Geometry: final body of the model. Coordinates: model frame, mm. Face numbers are marked on the shaded views. A direction names the side the tool comes from. Coordinates: 2 decimals unless noted, no trailing zeros. Order: outer loops, then holes, each group sorted by start corner. A loop starts at its lowest first (then second) coordinate and runs counter-clockwise, first axis right, second up. Notation, with made-up numbers: (15, 42) - (24, 42) arc R15 cw to (24, 65) - close; hole circle Ø4 at (-2, 85.5). An arc over 180 degrees is marked (long way). Use one line per item in the form item = value. Start each with the question number.
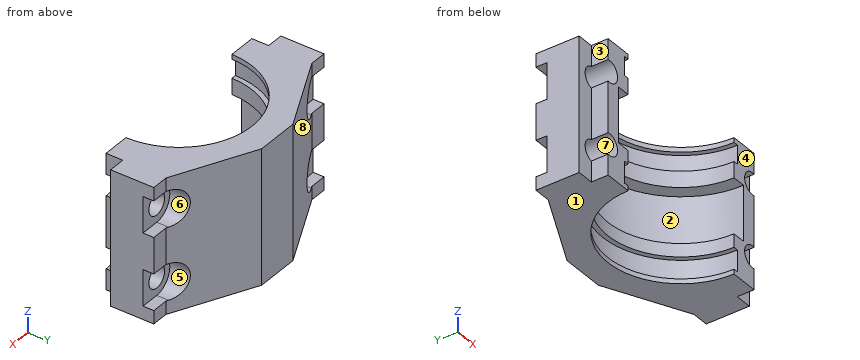
```python
from build123d import *

# Parameters (mm, degrees)
Y_KSEKLIK_EKSTR_ZYON1_DEPTH = 28
KES_EKSTR_ZYON1_DEPTH       = 7.81
KES_EKSTR_ZYON2_DEPTH       = 23
KES_EKSTR_ZYON3_DEPTH       = 9
KES_EKSTR_ZYON4_DEPTH       = 9
KES_EKSTR_ZYON5_DEPTH       = 4.5
IZIM7_R                     = 4.5
KES_EKSTR_ZYON6_DEPTH       = 21.5


with BuildPart() as part:
    # izim1 → Y_kseklik-Ekstr_zyon1 (new body, symmetric)
    with BuildSketch(Plane.XY):
        with BuildLine():
            Line((9, 0), (-9, 0))
            Line((-9, 0), (-42, -16))
            Line((-42, -16), (-49, -16))
            Line((-49, -16), (-49, -34))
            Line((-49, -34), (-42, -34))
            Line((-42, -34), (-42, -41))
            Line((-42, -41), (-30.5, -41))
            ThreePointArc((-30.5, -41), (0, -10.5), (30.5, -41))
            Line((30.5, -41), (42, -41))
            Line((42, -41), (42, -34))
            Line((42, -34), (49, -34))
            Line((49, -34), (49, -16))
            Line((49, -16), (42, -16))
            Line((42, -16), (9, 0))
        make_face()
    extrude(amount=Y_KSEKLIK_EKSTR_ZYON1_DEPTH, both=True)

    # izim2 → Kes-Ekstr_zyon1 (cut)
    with BuildSketch(Plane.XY.offset(26)):
        with BuildLine():
            Line((-32.5, -41), (32.5, -41))
            ThreePointArc((32.5, -41), (0, -8.5), (-32.5, -41))
        make_face()
    extrude(amount=-KES_EKSTR_ZYON1_DEPTH, mode=Mode.SUBTRACT)

    # izim3 → Kes-Ekstr_zyon2 (cut)
    with BuildSketch(Plane.XY.offset(11.5)):
        with BuildLine():
            Line((-36, -41), (36, -41))
            ThreePointArc((36, -41), (0, -5), (-36, -41))
        make_face()
    extrude(amount=-KES_EKSTR_ZYON2_DEPTH, mode=Mode.SUBTRACT)

    # izim4 → Kes-Ekstr_zyon3 (cut)
    with BuildSketch(Plane.XY.offset(-17)):
        with BuildLine():
            Line((-32.5, -41), (32.5, -41))
            ThreePointArc((32.5, -41), (0, -8.5), (-32.5, -41))
        make_face()
    extrude(amount=-KES_EKSTR_ZYON3_DEPTH, mode=Mode.SUBTRACT)

    # izim5 → Kes-Ekstr_zyon4 (cut)
    with BuildSketch(Plane(origin=(0, -16, 0), x_dir=(1, 0, 0), z_dir=(0, 1, 0))):
        with BuildLine():
            Line((41.09, -7.5), (49, -7.5))
            Line((49, -7.5), (49, -22.5))
            Line((49, -22.5), (41.09, -22.5))
            ThreePointArc((41.09, -22.5), (33.59, -15), (41.09, -7.5))
        make_face()
        with BuildLine():
            Line((41.09, 22.5), (49, 22.5))
            Line((49, 22.5), (49, 7.5))
            Line((49, 7.5), (41.09, 7.5))
            ThreePointArc((41.09, 7.5), (33.59, 15), (41.09, 22.5))
        make_face()
    kes_ekstr_zyon4 = extrude(amount=KES_EKSTR_ZYON4_DEPTH, mode=Mode.SUBTRACT)

    # izim5_2 → Kes-Ekstr_zyon5 (cut)
    with BuildSketch(Plane(origin=(0, -16, 0), x_dir=(1, 0, 0), z_dir=(0, 1, 0))):
        with BuildLine():
            Line((41.09, -7.5), (49, -7.5))
            Line((49, -7.5), (49, -22.5))
            Line((49, -22.5), (41.09, -22.5))
            ThreePointArc((41.09, -22.5), (33.59, -15), (41.09, -7.5))
        make_face()
        with BuildLine():
            Line((41.09, 22.5), (49, 22.5))
            Line((49, 22.5), (49, 7.5))
            Line((49, 7.5), (41.09, 7.5))
            ThreePointArc((41.09, 7.5), (33.59, 15), (41.09, 22.5))
        make_face()
    kes_ekstr_zyon5 = extrude(amount=-KES_EKSTR_ZYON5_DEPTH, mode=Mode.SUBTRACT)

    # Aynalama1: Kes-Ekstr_zyon4, Kes-Ekstr_zyon5 across plane
    add(kes_ekstr_zyon4.mirror(Plane(origin=(0, 0, 0), x_dir=(0, 0, 1), z_dir=(1, 0, 0))), mode=Mode.SUBTRACT)
    add(kes_ekstr_zyon5.mirror(Plane(origin=(0, 0, 0), x_dir=(0, 0, 1), z_dir=(1, 0, 0))), mode=Mode.SUBTRACT)

    # izim7 → Kes-Ekstr_zyon6 (cut, through all)
    with BuildSketch(Plane(origin=(0, -20.5, 0), x_dir=(1, 0, 0), z_dir=(0, 1, 0))):
        with Locations((-41.09, -15)):
            Circle(IZIM7_R)
        with Locations((-41.09, 15)):
            Circle(IZIM7_R)
    kes_ekstr_zyon6 = extrude(amount=-KES_EKSTR_ZYON6_DEPTH, mode=Mode.SUBTRACT)

    # Aynalama2: Kes-Ekstr_zyon6 across plane
    add(kes_ekstr_zyon6.mirror(Plane(origin=(0, 0, 0), x_dir=(0, 0, 1), z_dir=(1, 0, 0))), mode=Mode.SUBTRACT)


solid = part.part
```
(1) Material intervals for L1, parallel to Z at x = 41.09, y = -33.25; L2, parallel to X at y = -30, z = 15; L3, parallel to X at y = -27.5, z = 13, sorted ascending. Write a range as from..to.
(2) Draft query along X for the marked faces 6, 7 and 8. Return one class per face: released by +X, released by -X, zero draft, split by the parting line, or undercut.
(3) Cut plane C-C on z = -23.5. Return the cut outline in (x, y), plus the area to 3 significant figures.
(4) Cut plane A-A on z = 13. Return the cut outline in (x, y), plus the area to 3 significant figures.
(5) Cut plane B-B on x = 0. Return the cut outline in (y, z).
(6) Cut plane D-D on z = -16. Return the cut outline in (x, y), plus the area to 3 significant figures.
(7) Contact query for flat-ended pins moving along their axis: pin 1 Ø3 at (x, z) = (-45.5, 24.5) entering from +Y; pin 2 Ø2 at (y, z) = (-35.5, 9) entering from -X; pin 3 Ø7.5 at (y, z) = (-36.5, -1) entering from -X; pin 4 Ø18 at (x, y) = (-13, -29) entering from -Z. Output: stop coordinate, or through.
(8) Set-up query: the marked faces 1, 2, 3, 4 and 5. Return all of +Z, -Z, +X, -X, +Y, -Y with unobstructed straight access to the full face (end or side cutting, diameter ignored); none if empty.
Check sheet entries:
q1.L1 = -28..-19.5, -10.5..10.5, 19.5..28
q1.L2 = -49..-45.59, -36.59..-28.45, 28.45..36.59, 45.59..49
q1.L3 = -49..-45.12, -37.06..-27.35, 27.35..37.06, 45.12..49
q2.face_6 = released by +X
q2.face_7 = undercut
q2.face_8 = released by -X
q3.outline = (-49, -34) - (-42, -34) - (-42, -41) - (-32.5, -41) arc R32.5 cw to (32.5, -41) - (42, -41) - (42, -34) - (49, -34) - (49, -16) - (42, -16) - (9, 0) - (-9, 0) - (-42, -16) - (-49, -16) - close
q3.area = 1,510 mm^2
q4.outline = (-49, -34) - (-45.12, -34) - (-45.12, -20.5) - (-49, -20.5) - close; (-37.06, -41) - (-30.5, -41) arc R30.5 cw to (30.5, -41) - (37.06, -41) - (37.06, -20.5) - (33.86, -20.5) - (33.86, -12.05) - (9, 0) - (-9, 0) - (-33.86, -12.05) - (-33.86, -20.5) - (-37.06, -20.5) - close; (45.12, -34) - (49, -34) - (49, -20.5) - (45.12, -20.5) - close
q4.area = 1,250 mm^2
q5.outline = (-10.5, -28) - (0, -28) - (0, 28) - (-10.5, 28) - (-10.5, 26) - (-8.5, 26) - (-8.5, 18.19) - (-10.5, 18.19) - (-10.5, 11.5) - (-5, 11.5) - (-5, -11.5) - (-10.5, -11.5) - (-10.5, -17) - (-8.5, -17) - (-8.5, -26) - (-10.5, -26) - close
q6.outline = (-49, -34) - (-45.48, -34) - (-45.48, -20.5) - (-49, -20.5) - close; (-36.7, -41) - (-30.5, -41) arc R30.5 cw to (30.5, -41) - (36.7, -41) - (36.7, -20.5) - (33.66, -20.5) - (33.66, -11.95) - (9, 0) - (-9, 0) - (-33.66, -11.95) - (-33.66, -20.5) - (-36.7, -20.5) - close; (45.48, -34) - (49, -34) - (49, -20.5) - (45.48, -20.5) - close
q6.area = 1,220 mm^2
q7.pin_1 = -16
q7.pin_2 = -42
q7.pin_3 = -49
q7.pin_4 = through
q8.face_1 = -Z, +X, -X, +Y, -Y
q8.face_2 = -Y
q8.face_3 = +Z, -Z, -X, -Y
q8.face_4 = +Z, -Z, +X, -X, -Y
q8.face_5 = +X, +Y
